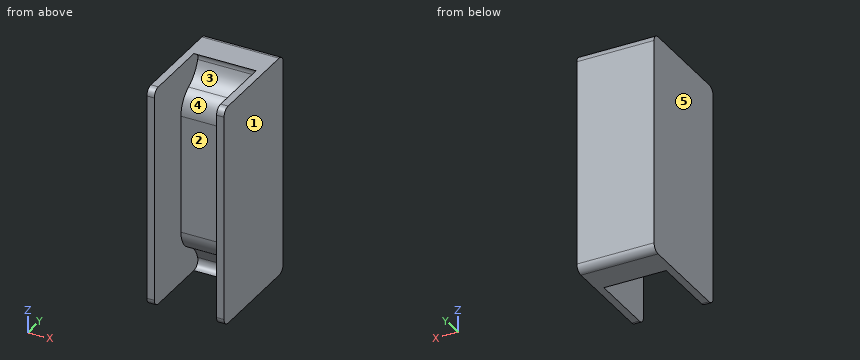
from build123d import *

# Parameters (mm, degrees)
RESSALTO_EXTRUS_O2_DEPTH = 25
RESSALTO_EXTRUS_O3_DEPTH = 3
RESSALTO_EXTRUS_O4_DEPTH = 3


with BuildPart() as part:
    # Esboço2 → Ressalto-extrusão2 (new body)
    with BuildSketch(Plane(origin=(0, 0, 0), x_dir=(0, 0, -1), z_dir=(1, 0, 0))):
        with BuildLine():
            Line((2.90159992, -0.062465938), (-35.09840008, -0.062465938))
            Line((-35.09840008, -0.062465938), (-39.886084903, -0.062465938))
            ThreePointArc((-39.886084903, -0.062465938), (-45.202180234, 1.467638524), (-48.891439328, 5.589707975))
            ThreePointArc((-48.891439328, 5.589707975), (-52.096536948, 9.772081499), (-56.69840008, 12.338743681))
            ThreePointArc((-56.69840008, 12.338743681), (-59.373224015, 11.895603401), (-60.59840008, 9.476926077))
            Line((-60.59840008, 9.476926077), (-60.59840008, 20.976926077))
            ThreePointArc((-60.59840008, 20.976926077), (-59.719720424, 23.09824642), (-57.59840008, 23.976926077))
            Line((-57.59840008, 23.976926077), (25.40159992, 23.976926077))
            ThreePointArc((25.40159992, 23.976926077), (27.522920263, 23.09824642), (28.40159992, 20.976926077))
            Line((28.40159992, 20.976926077), (28.40159992, 9.476926077))
            ThreePointArc((28.40159992, 9.476926077), (27.176423855, 11.895603401), (24.50159992, 12.338743681))
            ThreePointArc((24.50159992, 12.338743681), (19.899736788, 9.772081499), (16.694639168, 5.589707975))
            ThreePointArc((16.694639168, 5.589707975), (13.005380073, 1.467638524), (7.689284743, -0.062465938))
            Line((7.689284743, -0.062465938), (2.90159992, -0.062465938))
        make_face()
    extrude(amount=RESSALTO_EXTRUS_O2_DEPTH)

    # Esboço3 → Ressalto-extrusão3 (add)
    with BuildSketch(Plane.ZY):
        with BuildLine():
            Line((60.59840008, 15.226926077), (60.59840008, 20.976926077))
            ThreePointArc((60.59840008, 20.976926077), (59.719720424, 23.09824642), (57.59840008, 23.976926077))
            Line((57.59840008, 23.976926077), (16.09840008, 23.976926077))
            Line((16.09840008, 23.976926077), (-25.40159992, 23.976926077))
            ThreePointArc((-25.40159992, 23.976926077), (-27.522920263, 23.09824642), (-28.40159992, 20.976926077))
            Line((-28.40159992, 20.976926077), (-28.40159992, 15.226926077))
            Line((-28.40159992, 15.226926077), (-28.40159992, -16.773073923))
            ThreePointArc((-28.40159992, -16.773073923), (-27.522920263, -18.894394267), (-25.40159992, -19.773073923))
            Line((-25.40159992, -19.773073923), (57.59840008, -19.773073923))
            ThreePointArc((57.59840008, -19.773073923), (59.719720424, -18.894394267), (60.59840008, -16.773073923))
            Line((60.59840008, -16.773073923), (60.59840008, 15.226926077))
        make_face()
    extrude(amount=RESSALTO_EXTRUS_O3_DEPTH)

    # Esboço4 → Ressalto-extrusão4 (add)
    with BuildSketch(Plane(origin=(25, 0, 0), x_dir=(0, 0, -1), z_dir=(1, 0, 0))):
        with BuildLine():
            Line((-16.09840008, 23.976926077), (25.40159992, 23.976926077))
            ThreePointArc((25.40159992, 23.976926077), (27.522920263, 23.09824642), (28.40159992, 20.976926077))
            Line((28.40159992, 20.976926077), (28.40159992, 15.226926077))
            Line((28.40159992, 15.226926077), (28.40159992, -16.773073923))
            ThreePointArc((28.40159992, -16.773073923), (27.522920263, -18.894394267), (25.40159992, -19.773073923))
            Line((25.40159992, -19.773073923), (-57.59840008, -19.773073923))
            ThreePointArc((-57.59840008, -19.773073923), (-59.719720424, -18.894394267), (-60.59840008, -16.773073923))
            Line((-60.59840008, -16.773073923), (-60.59840008, 15.226926077))
            Line((-60.59840008, 15.226926077), (-60.59840008, 20.976926077))
            ThreePointArc((-60.59840008, 20.976926077), (-59.719720424, 23.09824642), (-57.59840008, 23.976926077))
            Line((-57.59840008, 23.976926077), (-16.09840008, 23.976926077))
        make_face()
    extrude(amount=RESSALTO_EXTRUS_O4_DEPTH)


solid = part.part
Work out the finished part from the listing and answer in its coordinate system (mm). Face numbers are marked on the shaded views. A direction names the side the tool comes from. Give positions to 0.01 mm unless a question says otherwise; leave off trailing zeros. Loops run counter-clockwise (first coordinate to the right, second up) from the corner with the lowest first, then second, coordinate; pieces in that order, holes last. Notation, with made-up numbers: (65, 80) -> (119, 80) arc R9 cw to (119, 92) -> close; hole circle Ø8 at (-36.5, 80). An arc over 180 degrees is marked (long way). Use a Markdown table: item, result. Add a question column.
1) The part is cut by section B-B, the plane z = 5. Determine the outline of the cut face in (x, y), plus the area to 3 significant figures.
2) Which of the six approach directions +Z, -Z, +X, -X, +Y, -Y give full straight-line access (tool end or side, diameter ignored) to the marked faces 1 and 2?
3) The part is cut by section D-D, the plane y = 11. Determine the outline of the cut face in (x, z), plus the area to 3 significant figures.
4) Consider line 1 along X through (y, z) = (4, -24.5); line 2 along Z through (x, y) = (16.5, 11); line 3 along Z through (x, y) = (3.5, 11.5). Determine where each line is inside the solid, lowest interval first.
5) The part is cut by section C-C, the plane x = 14.5. Determine the outline of the cut face in (y, z).
6) For a pull along Z with two mould halves and no side action, classify the marked faces 3, 4 and 5 as +Z half, -Z half, draft (parallel to the pull), parting line (faces both ways), or undercut.
7) The part is cut by section A-A, the plane y = -12. Determine the outline of the cut face in (x, z).
8) Each of these flat-tipped pins is pushed along its axis until it touches: P1, Ø10, axis at x = 12.5, z = 13.5, coming from the -Y side; P2, Ø2, axis at x = 8.5, y = 7, coming from the -Z side; P3, Ø10, axis at x = 17, y = -15.5, coming from the +Z side. Where does it stop, or does it pass through?
Reported:
| question | item | result |
|---|---|---|
| 1 | outline | (-3, -19.77) -> (0, -19.77) -> (0, -0.06) -> (25, -0.06) -> (25, -19.77) -> (28, -19.77) -> (28, 23.98) -> (-3, 23.98) -> close |
| 1 | area | 863 mm^2 |
| 2 | face 1 | +Z, -Z, +X, +Y, -Y |
| 2 | face 2 | +Z, -Z, -Y |
| 3 | outline | (-3, -28.4) -> (28, -28.4) -> (28, 60.6) -> (-3, 60.6) -> close; hole (0, -27.99) -> (25, -27.99) -> (25, -21.57) -> (0, -21.57) -> close; hole (0, 53.77) -> (25, 53.77) -> (25, 60.18) -> (0, 60.18) -> close |
| 3 | area | 2,440 mm^2 |
| 4 | line 1 | x = -3 to 0, 25 to 28 |
| 4 | line 2 | z = -28.4 to -27.99, -21.57 to 53.77, 60.18 to 60.6 |
| 4 | line 3 | z = -28.4 to -27.62, -22.46 to 54.66, 59.81 to 60.6 |
| 5 | outline | (-0.06, -7.69) arc R10 ccw to (5.59, -16.69) arc R13 cw to (12.34, -24.5) arc R3 cw to (9.48, -28.4) -> (20.98, -28.4) arc R3 ccw to (23.98, -25.4) -> (23.98, 57.6) arc R3 ccw to (20.98, 60.6) -> (9.48, 60.6) arc R3 cw to (12.34, 56.7) arc R13 cw to (5.59, 48.89) arc R10 ccw to (-0.06, 39.89) -> close |
| 6 | face 3 | undercut |
| 6 | face 4 | +Z half |
| 6 | face 5 | draft |
| 7 | outline | (-3, -28.4) -> (0, -28.4) -> (0, 60.6) -> (-3, 60.6) -> close; (25, -28.4) -> (28, -28.4) -> (28, 60.6) -> (25, 60.6) -> close |
| 8 | P1 | stops at y = -0.06 |
| 8 | P2 | stops at z = -18.2 |
| 8 | P3 | passes through |
